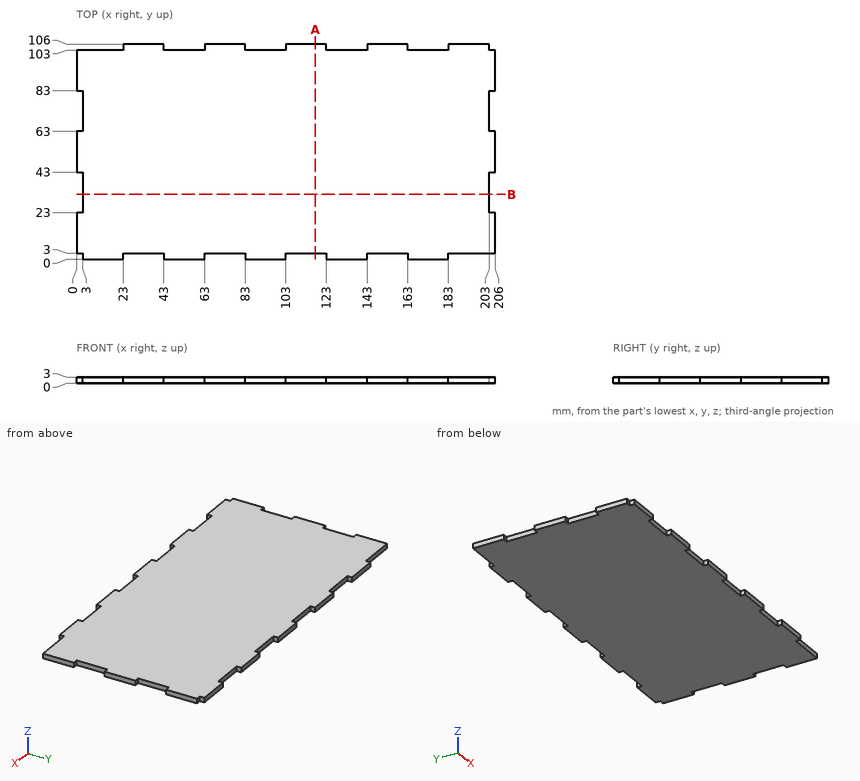
Can you work these out from the drawing? Everything is in mm from the part's minimum corner. Give positions to 0.01 mm unless a question says otherwise; leave off trailing zeros. Order: outer loops, then holes, each group sorted by start corner. A loop starts at its lowest first (then second) coordinate and runs counter-clockwise, first axis right, second up. Notation, with made-up numbers: M 36,76.5 L 68,76.5 A10 cw 68,89.5 Z; hole C -6,46 d7. An arc over 180 degrees is marked long. One line per item, written item: value.
Item 1: If we section it at B-B on y = 32: Write out the boundary of the cut face in (x, z), and give its area (3 significant figures).
Verdict:
outline: M 3,0 L 203,0 L 203,3 L 3,3 Z
area: 600 mm2
Item 2: Please list where these lines run through material, in increasing order: line 1 (X direction, y = 28.5, z = 1.95); line 2 (Y direction, x = 189.5, z = 1.7); line 3 (Y direction, x = 62, z = 0.25).
Verdict:
line 1: 3 to 203
line 2: 3 to 106
line 3: 0 to 103
Item 3: If we section it at A-A on x = 117.5: Write out the boundary of the cut face in (y, z), and give its area (3 significant figures).
Verdict:
outline: M 3,0 L 106,0 L 106,3 L 3,3 Z
area: 309 mm2
Item 4: For pin 1 (0.9 mm diameter, centred on x = 2, z = 1.5, fed in from -Y); pin 2 (1.5 mm diameter, centred on x = 16, z = 2, fed in from +Y); pin 3 (1.5 mm diameter, centred on y = 2, z = 1.5, fed in from +X), each with a flat end and sliding along its axis, tell me the tip position at first contact or that it passes through.
Verdict:
pin 1: y = 3
pin 2: y = 103
pin 3: x = 183
